Input: part model. Units: mm. Frame: model coordinates. Face numbers are marked on the shaded views. A direction names the side the tool comes from. Give positions to 0.01 mm unless a question says otherwise; leave off trailing zeros. Loops run counter-clockwise (first coordinate to the right, second up) from the corner with the lowest first, then second, coordinate; pieces in that order, holes last.
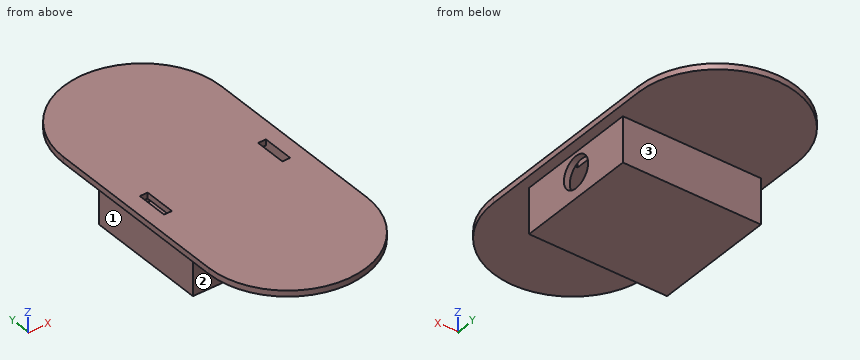
from build123d import *

# Parameters (mm, degrees)
F1_DEPTH  = 4.7625
F2_W      = 111.125
F2_H      = 98.425
F2_W_2    = 101.6
F2_H_2    = 88.9
F3_DEPTH  = 31.75
F5_D      = 25.4
F5_DEPTH  = 50.8
F6_W      = 6.35
F6_H      = 25.4
F7_DEPTH  = 4.7625
F9_W      = 111.125
F9_H      = 98.425
F10_DEPTH = 4.7625


with BuildPart() as f1:
    # F0 (on Top) → F1 (new body)
    with BuildSketch(Plane.XY):
        with BuildLine():
            ThreePointArc((-63.5, -76.2), (0, -139.7), (63.5, -76.2))
            Line((63.5, -76.2), (63.5, 76.2))
            ThreePointArc((63.5, 76.2), (0, 139.7), (-63.5, 76.2))
            Line((-63.5, 76.2), (-63.5, -76.2))
        make_face()
    extrude(amount=F1_DEPTH)

    # F2 (on face) → F3 (join)
    with BuildSketch(Plane(origin=(0, 0, 0), x_dir=(1, 0, 0), z_dir=(0, 0, -1))):
        Rectangle(F2_W, F2_H)
        Rectangle(F2_W_2, F2_H_2, mode=Mode.SUBTRACT)
    extrude(amount=F3_DEPTH)

    # F5
    with Locations(Plane.YZ.offset(55.5625)):
        with Locations((0, -15.875)):
            Hole(F5_D / 2, depth=F5_DEPTH)

    # F6 (on face) → F7 (cut)
    with BuildSketch(Plane.XY.offset(4.7625)):
        with Locations((47.625, 0)):
            Rectangle(F6_W, F6_H)
        with Locations((-47.625, 0)):
            Rectangle(F6_W, F6_H)
    extrude(amount=-F7_DEPTH, mode=Mode.SUBTRACT)

    # F9 (on offset) → F10 (join)
    with BuildSketch(Plane.XY.offset(-31.75)):
        Rectangle(F9_W, F9_H)
    extrude(amount=-F10_DEPTH)


solid = f1.part
(1) Reachability of the marked faces 1, 2 and 3 from +Z, -Z, +X, -X, +Y, -Y: full face, straight path, thin tool, end or side. Return the list, or none.
Values follow:
face 1: -Z, -X, +Y, -Y
face 2: -Z, +X, -X, -Y
face 3: -Z, +X, -X, +Y
(2) Cut plane B-B (y = 0). Count the separate pieces of the cut face and the enclosed holes in it, and give its area (3 significant figures).
Values follow:
separate pieces: 3
enclosed holes: 0
area: 1,260 mm2
(3) Cut plane C-C (z = -21). Return the cut outline in (x, y).
Values follow:
outline: (-55.56, -49.21) - (55.56, -49.21) - (55.56, -11.62) - (50.8, -11.62) - (50.8, -44.45) - (-50.8, -44.45) - (-50.8, 44.45) - (50.8, 44.45) - (50.8, 11.62) - (55.56, 11.62) - (55.56, 49.21) - (-55.56, 49.21) - close
(4) Pin query (flat end, axial travel): pin 1 Ø18.5 at (y, z) = (-24, -20) entering from +X; pin 2 Ø16 at (x, z) = (14.5, -14.5) entering from -Y; pin 3 Ø4 at (x, z) = (48, 2) entering from +Y (3 decimals). Return the tip coordinate at first contact, or that it passes through.
Values follow:
pin 1: stops at x = 55.56
pin 2: stops at y = -49.21
pin 3: stops at y = 119.975
(5) Cut plane A-A (x = 0). Return the cut outline in (y, z).
Values follow:
outline: (-139.7, 0) - (-49.21, 0) - (-49.21, -36.51) - (49.21, -36.51) - (49.21, 0) - (139.7, 0) - (139.7, 4.76) - (-139.7, 4.76) - close; hole (-44.45, -31.75) - (44.45, -31.75) - (44.45, 0) - (-44.45, 0) - close
(6) Cut plane D-D (y = -67.5). Return the cut outline in (x, z), and give its area (3 significant figures).
Values follow:
outline: (-63.5, 0) - (63.5, 0) - (63.5, 4.76) - (-63.5, 4.76) - close
area: 605 mm2
(7) Ray query, probe 1 along X at (y, z) = (23.5, -16.5); probe 2 along Y at (x, z) = (46.5, -19); probe 3 along Z at (x, y) = (54.4, 0) (1 decimal). Return the intervals inside material, ascending.
Values follow:
probe 1: x = -55.56 to -50.8, 50.8 to 55.56
probe 2: y = -49.21 to -44.45, 44.45 to 49.21
probe 3: z = -36.5 to -28.6, -3.2 to 4.8
